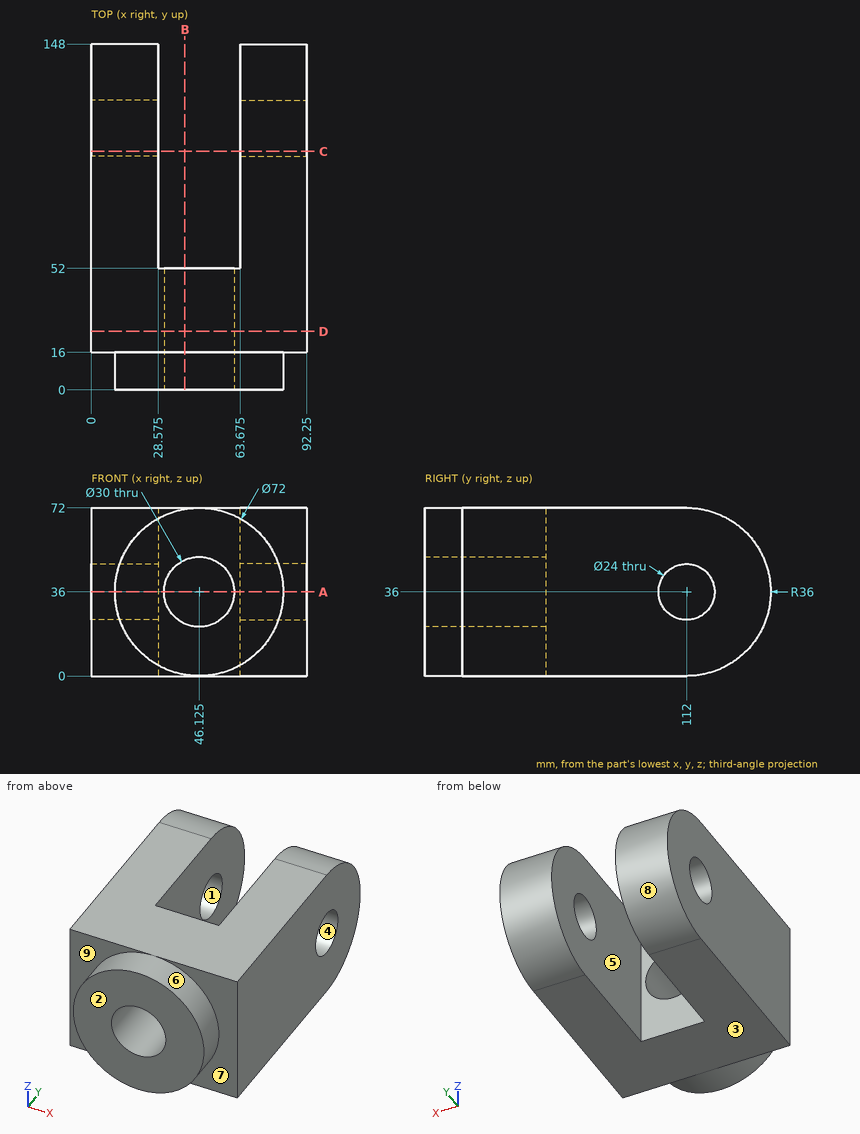
Design review of the part shown in the three views and the two pictorial views. Dimensions are in mm from the part's minimum x, y and z. A direction names the side the tool comes from. Round coordinates to 2 decimals unless told otherwise and drop trailing zeros. Write each loop counter-clockwise with the first axis right and the second up, starting at its lowest first coordinate (ties: lowest second). Pieces come first, ordered by that corner, then holes.
Item 1: Consider section A-A on z = 36. Give the boundary of the cut face in (x, y) (3 decimals).
Item 2: For the marked faces 5, 6, 7, 8 and 9, list the 3-axis set-ups (+Z, -Z, +X, -X, +Y, -Y) from which the entire face can be reached by the end or side of a thin tool; tool diameter is ignored.
Item 3: Draft analysis for pull direction Y (two halves, no side actions). For the marked faces 1, 2, 3 and 4, state which applies: released by +Y, released by -Y, zero draft, split by the parting line, or undercut.
Item 4: Consider section C-C on y = 102. Give the boundary of the cut face in (x, z) (3 decimals).
Item 5: Consider section D-D on y = 25. Give the boundary of the cut face in (x, z) (3 decimals), and give its area (3 significant figures).
Item 6: For pin 1 Ø2 at (x, z) = (64.5, 35) entering from -Y; pin 2 Ø8 at (x, z) = (83, 54) entering from +Y; pin 3 Ø2 at (x, y) = (12.5, 123) entering from +Z; pin 4 Ø10.5 at (x, z) = (40.5, 46) entering from +Y, all flat-tipped, find the tip position at first contact; note any pin that passes through.
Item 7: Consider section B-B on x = 40. Give the boundary of the cut face in (y, z), and give its area (3 significant figures).
Item 8: Wall thickness on L1, parallel to Y at x = 85.75, z = 36; L2, parallel to X at y = 107, z = 25 (3 decimals); L3, parallel to X at y = 15, z = 36 (3 decimals): over which ranges is each line inside the solid? List them lowest first.
Check values:
1. outline: (0, 16) - (10.125, 16) - (10.125, 0) - (31.125, 0) - (31.125, 52) - (28.575, 52) - (28.575, 100) - (0, 100) - close; (0, 124) - (28.575, 124) - (28.575, 148) - (0, 148) - close; (61.125, 0) - (82.125, 0) - (82.125, 16) - (92.25, 16) - (92.25, 100) - (63.675, 100) - (63.675, 52) - (61.125, 52) - close; (63.675, 124) - (92.25, 124) - (92.25, 148) - (63.675, 148) - close
2. face 5: +Z, -Z, +Y
2. face 6: -Y
2. face 7: +X, -Y
2. face 8: +X, -X, +Y
2. face 9: -X, -Y
3. face 1: undercut
3. face 2: released by -Y
3. face 3: zero draft
3. face 4: undercut
4. outline: (0, 0) - (28.575, 0) - (28.575, 29.367) - (0, 29.367) - close; (0, 42.633) - (28.575, 42.633) - (28.575, 72) - (0, 72) - close; (63.675, 0) - (92.25, 0) - (92.25, 29.367) - (63.675, 29.367) - close; (63.675, 42.633) - (92.25, 42.633) - (92.25, 72) - (63.675, 72) - close
5. outline: (0, 0) - (92.25, 0) - (92.25, 72) - (0, 72) - close; hole circle Ø30 at (46.125, 36)
5. area: 5,940 mm2
6. pin 1: stops at y = 0
6. pin 2: stops at y = 145.17
6. pin 3: stops at z = 70.58
6. pin 4: stops at y = 52
7. outline: (0, 0.52) - (16, 0.52) - (16, 0) - (52, 0) - (52, 22.31) - (0, 22.31) - close; (0, 49.69) - (52, 49.69) - (52, 72) - (16, 72) - (16, 71.48) - (0, 71.48) - close
7. area: 2,300 mm2
8. L1: y = 16 to 100, 124 to 148
8. L2: x = 0 to 28.575, 63.675 to 92.25
8. L3: x = 10.125 to 31.125, 61.125 to 82.125
